from build123d import *

# Parameters (mm, degrees)
SKETCH1_R      = 4.5
EXTRUDE1_DEPTH = 8


with BuildPart() as part:
    # Sketch1 → Extrude1 (new body)
    with BuildSketch(Plane.XY):
        with BuildLine():
            Line((-9, 0), (-9, -14.5))
            ThreePointArc((-9, -14.5), (-7.918317006, -16.806525496), (-5.453293424, -17.449764723))
            Line((-5.453293424, -17.449764723), (66.546706576, -4.105353488))
            ThreePointArc((66.546706576, -4.105353488), (68.306525496, -3.073905771), (69, -1.155588765))
            Line((69, -1.155588765), (69, 11.5))
            ThreePointArc((69, 11.5), (62.434509272, 20.164477169), (52.317074532, 16.1875))
            ThreePointArc((52.317074532, 16.1875), (46.854286329, 10.91971904), (39.512198751, 9))
            Line((39.512198751, 9), (0, 9))
            ThreePointArc((0, 9), (-6.363961031, 6.363961031), (-9, 0))
        make_face()
        Circle(SKETCH1_R, mode=Mode.SUBTRACT)
        with Locations((60, 11.5)):
            Circle(SKETCH1_R, mode=Mode.SUBTRACT)
    extrude(amount=EXTRUDE1_DEPTH)


solid = part.part
Source: CAD feature listing. Evaluate the final solid. Frame: model axes, mm. A direction names the side the tool comes from. Coordinates: 2 decimals unless noted, no trailing zeros. Order: outer loops, then holes, each group sorted by start corner. A loop starts at its lowest first (then second) coordinate and runs counter-clockwise, first axis right, second up. Notation, with made-up numbers: M 12.25,3.25 L 37.25,3.25 A33 ccw 37.25,39.25 Z; hole C 77.5,6 d7. An arc over 180 degrees is marked long. Write each question's results on one line, items separated by ' | '. Start each with the question number.
Item 1: Cut plane D-D (x = 19). Return loops of the section in (y, z).
Item 2: Set-up query: faces 1 (the face through (20, 9, 4)), 2 (the face through (29, 2, 0)). Return all of +Z, -Z, +X, -X, +Y, -Y with unobstructed straight access to the full face (end or side cutting, diameter ignored); none if empty.
Item 3: Line query: probe 1 along Y at (x, z) = (0, 5.25); probe 2 along Y at (x, z) = (60, 4.5); probe 3 along X at (y, z) = (14, 7.5). Output: solid intervals per line, ascending.
Item 4: Draft query along X for faces 3 (the face through (62.59, 20.12, 3.94)), 4 (the face through (64.16, 9.78, 3.94)), 5 (the face through (-9, -7, 4)), 6 (the face through (-0.59, 4.46, 3.94)). Return one class per face: pulls with the +X half, pulls with the -X half, needs draft (parallel to the pull), parting line crosses it, or undercut.
Item 5: First-contact query: pin 1 Ø2.5 at (x, z) = (16.5, 4) entering from +Y. Flat tip, straight axial feed; report the tip coordinate or a pass-through.
Item 6: Cut plane C-C (y = -3). Return loops of the section in (x, z).
Item 7: Cut plane B-B (z = 7). Return loops of the section in (x, y).
Item 8: Cut plane A-A (x = 61.5). Return loops of the section in (y, z), and give its area (3 significant figures).
Checked values:
1) outline: M -12.92,0 L 9,0 L 9,8 L -12.92,8 Z
2) face 1: +Z, -Z, -X, +Y | face 2: -Z, +X, -X, +Y, -Y
3) probe 1: y = -16.44 to -4.5, 4.5 to 9 | probe 2: y = -5.32 to 7, 16 to 20.5 | probe 3: x = 50.69 to 56.26, 63.74 to 68.65
4) face 3: parting line crosses it | face 4: undercut | face 5: pulls with the -X half | face 6: undercut
5) pin 1: stops at y = 9
6) outline: M -9,0 L -3.35,0 L -3.35,8 L -9,8 Z; M 3.35,0 L 68.37,0 L 68.37,8 L 3.35,8 Z
7) outline: M -9,-14.5 A3 ccw -5.45,-17.45 L 66.55,-4.11 A3 ccw 69,-1.16 L 69,11.5 A9 ccw 52.32,16.19 A15 cw 39.51,9 L 0,9 A9 ccw -9,0 Z; hole C 0,0 d9; hole C 60,11.5 d9
8) outline: M -5.04,0 L 7.26,0 L 7.26,8 L -5.04,8 Z; M 15.74,0 L 20.37,0 L 20.37,8 L 15.74,8 Z | area: 135 mm2
